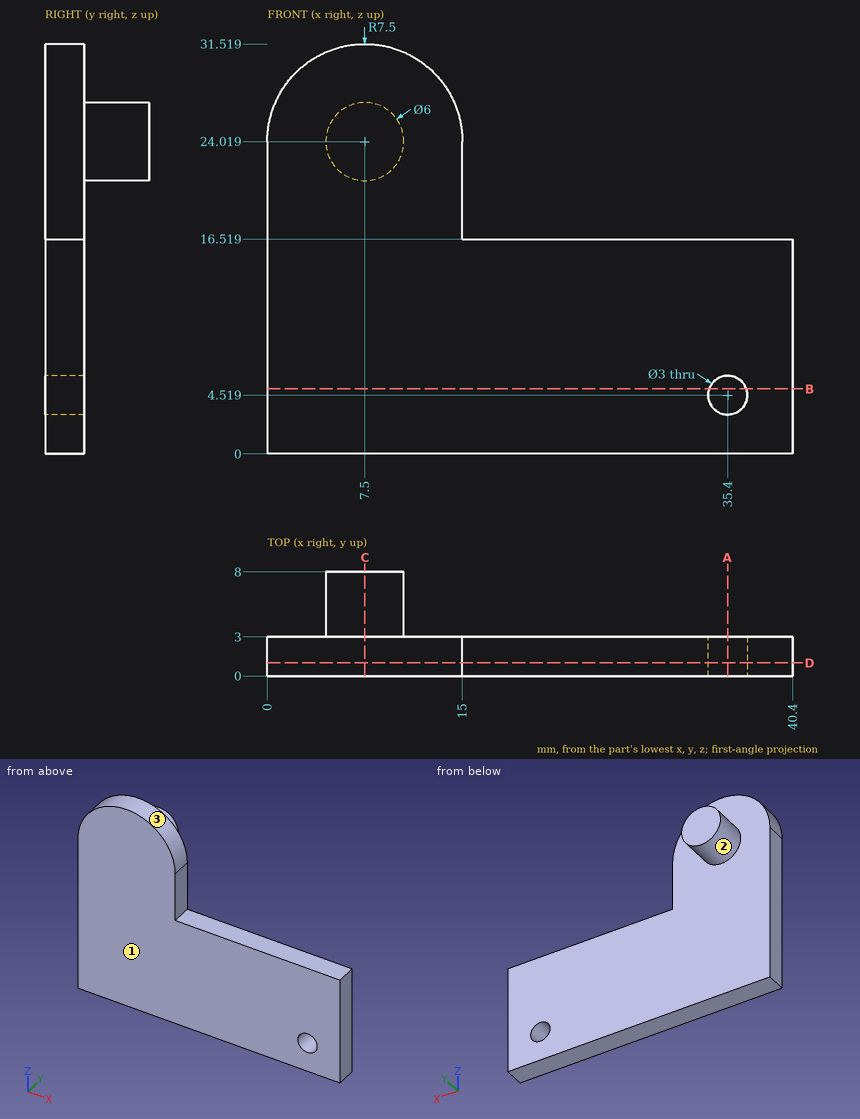
Print and shaded views of the part. All mm, measured from the part's lowest x, y and z. Give positions to 0.01 mm unless a question says otherwise; leave off trailing zeros. Write each loop counter-clockwise with the first axis right and the second up, starting at its lowest first coordinate (ties: lowest second). Pieces come first, ordered by that corner, then holes. Notation, with made-up numbers: (-32, 52.25) - (18, 52.25) arc R15 cw to (18, 66.25) - close; hole circle Ø3 at (-18, 8.5). An arc over 180 degrees is marked (long way). One line per question, with ' | ' between items. Start each with the question number.
(1) Slice it at B-B on z = 5. Write the cut outline in (x, y).
(2) Slice it at A-A on x = 35.4. Write the cut outline in (y, z).
(3) Pin check, flat tips, straight feed: P1, Ø2, axis at x = 18.5, z = 8, coming from the +Y side; P2, Ø4, axis at y = 5.5, z = 22, coming from the +X side; P3, Ø0.9, axis at y = 2, z = 19, coming from the +X side; P4, Ø1.8, axis at x = 35.4, z = 4.519, coming from the +Y side. Stop position of each tip, or through.
(4) Slice it at C-C on x = 7.5. Write the cut outline in (y, z), plus the area to 3 significant figures.
(5) Wall check: line 1 along Z through (x, y) = (35.4, 1.55); line 2 along Y through (x, z) = (7, 17.5); line 3 along X through (y, z) = (2.5, 21). Give the ranges that are in metal, low to high. Write a range as from..to.
(6) Slice it at D-D on y = 1. Write the cut outline in (x, z).
(7) Two-plate mould, pull along Z, no slides. Class the marked faces 1, 2 and 3: +Z half, -Z half, draft (parallel to the pull), parting line (faces both ways), or undercut.
Results below:
1) outline: (0, 0) - (33.98, 0) - (33.98, 3) - (0, 3) - close; (36.82, 0) - (40.4, 0) - (40.4, 3) - (36.82, 3) - close
2) outline: (0, 0) - (3, 0) - (3, 3.02) - (0, 3.02) - close; (0, 6.02) - (3, 6.02) - (3, 16.52) - (0, 16.52) - close
3) P1: y = 3 | P2: x = 10.5 | P3: x = 15 | P4: through
4) outline: (0, 0) - (3, 0) - (3, 21.02) - (8, 21.02) - (8, 27.02) - (3, 27.02) - (3, 31.52) - (0, 31.52) - close | area: 125 mm^2
5) line 1: 0..3.02, 6.02..16.52 | line 2: 0..3 | line 3: 0..15
6) outline: (0, 0) - (40.4, 0) - (40.4, 16.52) - (15, 16.52) - (15, 24.02) arc R7.5 ccw to (0, 24.02) - close; hole circle Ø3 at (35.4, 4.52)
7) face 1: draft | face 2: parting line | face 3: +Z half
